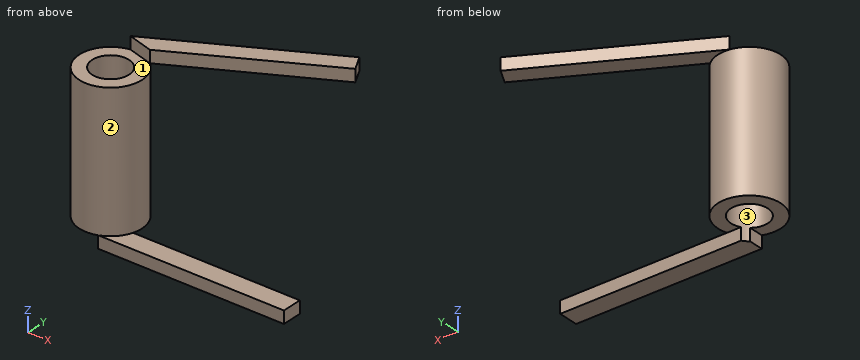
from build123d import *

# Parameters (mm, degrees)
SKETCH1_R      = 2.55
EXTRUDE1_DEPTH = 11
EXTRUDE2_DEPTH = 1
SKETCH3_W      = 15.099881368
SKETCH3_H      = 1.61958708
EXTRUDE3_DEPTH = 1
SKETCH4_R      = 1.5
EXTRUDE4_DEPTH = 13


with BuildPart() as part:
    # Sketch1 → Extrude1 (new body)
    with BuildSketch(Plane.XY):
        Circle(SKETCH1_R)
    extrude(amount=EXTRUDE1_DEPTH)

    # Sketch2 → Extrude2 (add)
    with BuildSketch(Plane.XY.offset(11)):
        Polygon((1.650889975, 1.943466565), (13.374427377, 8.212697839), (12.680705309, 9.509966398), (-0.390866423, 2.519865758), align=None)
    extrude(amount=EXTRUDE2_DEPTH)

    # Sketch3 → Extrude3 (add)
    with BuildSketch(Plane(origin=(0, 0, 0), x_dir=(-1, 0, 0), z_dir=(0, 0, -1))):
        with Locations((-8.442177906, -1.57901636)):
            Rectangle(SKETCH3_W, SKETCH3_H)
    extrude(amount=EXTRUDE3_DEPTH)

    # Sketch4 → Extrude4 (cut, through all)
    with BuildSketch(Plane.XY.offset(11)):
        Circle(SKETCH4_R)
    extrude(amount=-EXTRUDE4_DEPTH, mode=Mode.SUBTRACT)


solid = part.part
Part model, mm, in its own coordinate system. Face numbers are marked on the shaded views. Coordinates: 2 decimals unless noted, no trailing zeros. Order: outer loops, then holes, each group sorted by start corner. A loop starts at its lowest first (then second) coordinate and runs counter-clockwise, first axis right, second up.
(1) Slice it at A-A, the plane y = 0. Write the cut outline in (x, z), and give its area (3 significant figures).
Check sheet entries:
outline: (-2.55, 0) - (-1.5, 0) - (-1.5, 11) - (-2.55, 11) - close; (1.5, 0) - (2.55, 0) - (2.55, 11) - (1.5, 11) - close
area: 23.1 mm2
(2) Pin check, flat tips, straight feed: pin 1 Ø0.8 at (x, y) = (11, -1.5) entering from +Z; pin 2 Ø3 at (x, z) = (13.5, 9) entering from -Y; pin 3 Ø0.5 at (y, z) = (-2, -0.5) entering from -X; pin 4 Ø1.5 at (y, z) = (1.5, 9.5) entering from +X. Stop position of each tip, or through.
Check sheet entries:
pin 1: stops at z = 0
pin 2: passes through
pin 3: stops at x = 0.89
pin 4: stops at x = 2.44
(3) Slice it at D-D, the plane x = 4. Write the cut outline in (y, z).
Check sheet entries:
outline: (-2.39, -1) - (-0.77, -1) - (-0.77, 0) - (-2.39, 0) - close; (3.2, 11) - (4.87, 11) - (4.87, 12) - (3.2, 12) - close
(4) Probe L1, parallel to Y at x = 0, z = 4; L2, parallel to Z at x = 3.5, y = 3.75. List the from-to ranges inside material, lowest first.
Check sheet entries:
L1: y = -2.55 to -1.5, 1.5 to 2.55
L2: z = 11 to 12
(5) Slice it at C-C, the plane z = 9.25. Write the cut outline in (x, y).
Check sheet entries:
outline: circle Ø5.1 at (0, 0); hole circle Ø3 at (0, 0)
(6) Pull direction X, two halves, no side cores. Call the marked faces 1, 2 and 3: pulls with the +X half, pulls with the -X half, needs draft (parallel to the pull), parting line crosses it, or undercut.
Check sheet entries:
face 1: needs draft
face 2: parting line crosses it
face 3: undercut
(7) Slice it at B-B, the plane x = 0. Write the cut outline in (y, z).
Check sheet entries:
outline: (-2.55, 0) - (-1.5, 0) - (-1.5, 11) - (-2.55, 11) - close; (1.5, 0) - (2.55, 0) - (2.55, 11) - (2.73, 11) - (2.73, 12) - (2.41, 12) - (2.41, 11) - (1.5, 11) - close
